```python
from build123d import *

# Parameters (mm, degrees)
EXTRUDE_1_DEPTH     = 3
SKETCH_3_R          = 1.5
CUT_EXTRUDE_3_DEPTH = 5


with BuildPart() as part:
    # 草图1 → 凸台-拉伸1 (new body)
    with BuildSketch(Plane.XY):
        with BuildLine():
            Line((0, 0), (0, 60))
            ThreePointArc((0, 60), (3, 63), (6, 60))
            Line((6, 60), (6, 0))
            ThreePointArc((6, 0), (3, -3), (0, 0))
        make_face()
    extrude(amount=EXTRUDE_1_DEPTH)

    # 草图3 → 切除-拉伸3 (cut)
    with BuildSketch(Plane.XY):
        with Locations((3, 0)):
            Circle(SKETCH_3_R)
        with Locations((3, 60)):
            Circle(SKETCH_3_R)
        with Locations((3, 48)):
            Circle(SKETCH_3_R)
    extrude(amount=CUT_EXTRUDE_3_DEPTH, mode=Mode.SUBTRACT)


solid = part.part
```
Here's how the part is built. I have some questions about the finished solid (model axes, mm). Round coordinates to 2 decimals unless told otherwise and drop trailing zeros. Write each loop counter-clockwise with the first axis right and the second up, starting at its lowest first coordinate (ties: lowest second). Pieces come first, ordered by that corner, then holes.
Q1. If we section it at C-C on x = 3: Write out the boundary of the cut face in (y, z), plus the area to 3 significant figures.
Q2. If we section it at A-A on y = 48: Write out the boundary of the cut face in (x, z), plus the area to 3 significant figures.
Q3. Will these pins go through, and if not, where does the flat tip stop? P1, Ø1, axis at x = 5.5, z = 0.5, coming from the +Y side; P2, Ø3.5, axis at x = 3, y = 0, coming from the -Z side; P3, Ø1.5, axis at x = 5, z = 1, coming from the +Y side.
Q4. If we mould it in two halves opening along X, with no side actions, what happens to faces 1 (the cylindrical face through (3, -3, 1)), 2 (the cylindrical face through (2.675, 46.536, 1.479)), 3 (the flat face through (3, 30, 0)), 4 (the cylindrical face through (2.805, 61.487, 1.479))? For each: +X half, -X half, draft (parallel to the pull), parting line (faces both ways), or undercut.
Q5. Please list where these lines run through material, in increasing order: probe 1 along Y at (x, z) = (3, 1.1); probe 2 along X at (y, z) = (48, 2.15); probe 3 along X at (y, z) = (47, 1.45).
Q6. If we section it at B-B on z = 0.8: Write out the boundary of the cut face in (x, y).
Answer below:
1. outline: (-3, 0) - (-1.5, 0) - (-1.5, 3) - (-3, 3) - close; (1.5, 0) - (46.5, 0) - (46.5, 3) - (1.5, 3) - close; (49.5, 0) - (58.5, 0) - (58.5, 3) - (49.5, 3) - close; (61.5, 0) - (63, 0) - (63, 3) - (61.5, 3) - close
1. area: 171 mm2
2. outline: (0, 0) - (1.5, 0) - (1.5, 3) - (0, 3) - close; (4.5, 0) - (6, 0) - (6, 3) - (4.5, 3) - close
2. area: 9.00 mm2
3. P1: stops at y = 62.24
3. P2: stops at z = 0
3. P3: stops at y = 62.73
4. face 1: parting line
4. face 2: undercut
4. face 3: draft
4. face 4: undercut
5. probe 1: y = -3 to -1.5, 1.5 to 46.5, 49.5 to 58.5, 61.5 to 63
5. probe 2: x = 0 to 1.5, 4.5 to 6
5. probe 3: x = 0 to 1.88, 4.12 to 6
6. outline: (0, 0) arc R3 ccw to (6, 0) - (6, 60) arc R3 ccw to (0, 60) - close; hole circle Ø3 at (3, 0); hole circle Ø3 at (3, 48); hole circle Ø3 at (3, 60)
